from build123d import *

# Parameters (mm, degrees)
SKETCH1_W                      = 254
SKETCH1_H                      = 203.2
SKETCH1_R                      = 3.05
SKETCH1_W_2                    = 203.2
SKETCH1_H_2                    = 152.4
BOSS_EXTRUDE1_DEPTH            = 6.35
SKETCH2_R                      = 6.35
CUT_EXTRUDE1_DEPTH             = 3
CBORE_FOR_M5_SHCS1_D           = 5.5
CBORE_FOR_M5_SHCS1_CBORE_D     = 10
CBORE_FOR_M5_SHCS1_CBORE_DEPTH = 5


with BuildPart() as part:
    # Sketch1 → Boss-Extrude1 (new body)
    with BuildSketch(Plane(origin=(0, 0, 0), x_dir=(1, 0, 0), z_dir=(0, 1, 0))):
        with Locations((127, 101.6)):
            Rectangle(SKETCH1_W, SKETCH1_H)
        with Locations((12.7, 190.5)):
            Circle(SKETCH1_R, mode=Mode.SUBTRACT)
        with Locations((241.3, 190.5)):
            Circle(SKETCH1_R, mode=Mode.SUBTRACT)
        with Locations((241.3, 12.7)):
            Circle(SKETCH1_R, mode=Mode.SUBTRACT)
        with Locations((12.7, 12.7)):
            Circle(SKETCH1_R, mode=Mode.SUBTRACT)
        with Locations((127, 101.6)):
            Rectangle(SKETCH1_W_2, SKETCH1_H_2, mode=Mode.SUBTRACT)
    extrude(amount=BOSS_EXTRUDE1_DEPTH)

    # Sketch2 → Cut-Extrude1 (cut)
    with BuildSketch(Plane(origin=(0, 6.35, 0), x_dir=(1, 0, 0), z_dir=(0, 1, 0))):
        with Locations((12.7, 190.5)):
            Circle(SKETCH2_R)
        with Locations((241.3, 190.5)):
            Circle(SKETCH2_R)
        with Locations((241.3, 12.7)):
            Circle(SKETCH2_R)
        with Locations((12.7, 12.7)):
            Circle(SKETCH2_R)
    extrude(amount=-CUT_EXTRUDE1_DEPTH, mode=Mode.SUBTRACT)

    # CBORE for M5 SHCS1 (through all)
    with Locations(Plane(origin=(0, 6.35, 0), x_dir=(1, 0, 0), z_dir=(0, 1, 0))):
        with Locations((246.38, 76.2), (246.38, 127), (7.62, 76.2), (7.62, 127)):
            CounterBoreHole(CBORE_FOR_M5_SHCS1_D / 2, CBORE_FOR_M5_SHCS1_CBORE_D / 2, CBORE_FOR_M5_SHCS1_CBORE_DEPTH)


solid = part.part
Check sheet for the modelled part. Datum: model origin and axes. Units: mm. A direction names the side the tool comes from. Give positions to 0.01 mm unless a question says otherwise; leave off trailing zeros. Write each loop counter-clockwise with the first axis right and the second up, starting at its lowest first coordinate (ties: lowest second). Pieces come first, ordered by that corner, then holes. Notation, with made-up numbers: (-7, 71) -> (11, 71) arc R27 ccw to (11, 88) -> close; hole circle Ø7 at (37.25, 16.25). An arc over 180 degrees is marked (long way). One line per item, written item: value. Start each with the question number.
Item 1: Section check A-A on z = -12.7. Record the cut outline in (x, y).
Item 2: Tool access check on faces 3 (the flat face through (249, 1.35, -125)), 4 (the flat face through (125, 0, -193)), 5 (the flat face through (228.6, 3, -101)). Record the directions out of +Z, -Z, +X, -X, +Y, -Y that give a thin tool (end or side, any length) a straight path to the whole face; none if there is none.
Item 3: Section check C-C on x = 125. Record the cut outline in (y, z).
Item 4: Gauge pin test, flat ends, axial feed: pin 1 (10 mm diameter, centred on x = 12.7, z = -190.5, fed in from +Y); pin 2 (5 mm diameter, centred on x = 7.62, z = -127, fed in from +Y). Record the tip position at first contact, or that the pin passes through.
Item 5: Draft check along Z on faces 1 (the flat face through (10, 1.35, -125)), 2 (the flat face through (254, 3, -100)). Enter one of: +Z half, -Z half, draft (parallel to the pull), parting line (faces both ways), or undercut.
Item 6: Material ranges on probe 1 along X at (y, z) = (4.9, -12.7); probe 2 along Z at (x, y) = (12.7, 1.8); probe 3 along X at (y, z) = (3.45, -127), recorded low to high. Write a range as from..to.
Item 7: Section check B-B on z = -76.2. Record the cut outline in (x, y).
Item 8: Section check D-D on z = -103. Record the cut outline in (x, y).
Results list:
1. outline: (0, 0) -> (9.65, 0) -> (9.65, 3.35) -> (6.35, 3.35) -> (6.35, 6.35) -> (0, 6.35) -> close; (15.75, 0) -> (238.25, 0) -> (238.25, 3.35) -> (234.95, 3.35) -> (234.95, 6.35) -> (19.05, 6.35) -> (19.05, 3.35) -> (15.75, 3.35) -> close; (244.35, 0) -> (254, 0) -> (254, 6.35) -> (247.65, 6.35) -> (247.65, 3.35) -> (244.35, 3.35) -> close
2. face 3: +Y
2. face 4: +Z, -Z, +X, -X, -Y
2. face 5: +Y, -Y
3. outline: (0, -203.2) -> (6.35, -203.2) -> (6.35, -177.8) -> (0, -177.8) -> close; (0, -25.4) -> (6.35, -25.4) -> (6.35, 0) -> (0, 0) -> close
4. pin 1: y = 3.35
4. pin 2: through
5. face 1: undercut
5. face 2: draft
6. probe 1: 0..6.35, 19.05..234.95, 247.65..254
6. probe 2: -203.2..-193.55, -187.45..-15.75, -9.65..0
6. probe 3: 0..2.62, 12.62..25.4, 228.6..241.38, 251.38..254
7. outline: (0, 0) -> (4.87, 0) -> (4.87, 1.35) -> (2.62, 1.35) -> (2.62, 6.35) -> (0, 6.35) -> close; (10.37, 0) -> (25.4, 0) -> (25.4, 6.35) -> (12.62, 6.35) -> (12.62, 1.35) -> (10.37, 1.35) -> close; (228.6, 0) -> (243.63, 0) -> (243.63, 1.35) -> (241.38, 1.35) -> (241.38, 6.35) -> (228.6, 6.35) -> close; (249.13, 0) -> (254, 0) -> (254, 6.35) -> (251.38, 6.35) -> (251.38, 1.35) -> (249.13, 1.35) -> close
8. outline: (0, 0) -> (25.4, 0) -> (25.4, 6.35) -> (0, 6.35) -> close; (228.6, 0) -> (254, 0) -> (254, 6.35) -> (228.6, 6.35) -> close
